Autodesk Inventor part; units mm, degrees
ref_plane "YZ Plane" through (0, 0, 0) normal (1, 0, 0) x (0, 1, 0)
ref_plane "XZ Plane" through (0, 0, 0) normal (0, 1, 0) x (-1, 0, 0)
ref_plane "XY Plane" through (0, 0, 0) normal (0, 0, 1) x (1, 0, 0)
sketch "Sketch1" plane through (0, 0, 0) normal (1, 0, 0) x (0, 1, 0)
  line L0 (0, 0) -> (50.8, 0)
  line L1 (50.8, 0) -> (50.8, -25.4)
  line L2 (50.8, -25.4) -> (0, -25.4)
  line L3 (0, -25.4) -> (0, 0)
  line L4 (2.54, -2.54) -> (48.26, -2.54)
  line L5 (48.26, -2.54) -> (48.26, -22.86)
  line L6 (48.26, -22.86) -> (2.54, -22.86)
  line L7 (2.54, -22.86) -> (2.54, -2.54)
  dimension "d0" = 50.8
  dimension "d1" = 25.4
  dimension "d2" = 45.72
  dimension "d3" = 20.32
  dimension "d4" = 2.54
  dimension "d5" = 2.54
extrude "Extrusion1" add sketch "Sketch1" along normal blind 76.2
sketch "Sketch2" plane through (0, 50.8, 0) normal (0, 1, 0) x (1, 0, 0)
  line L0 (0, 0) -> (0, 25.4)
  line L1 (0, 0) -> (76.2, 0)
  line L2 (76.2, 25.4) -> (76.2, 0)
  line L3 (0, 25.4) -> (76.2, 25.4)
  point P0 (12.7, 12.7)
  point P1 (38.1, 12.7)
  point P2 (63.5, 12.7)
  dimension "d8" = 12.7
  dimension "d9" = 12.7
  dimension "d10" = 12.7
  dimension "d11" = 12.7
  dimension "d12" = 38.1
  dimension "d13" = 63.5
hole "Hole1" at (12.7, 50.8, -12.7) at (38.1, 50.8, -12.7) at (63.5, 50.8, -12.7) direction (0, -1, 0) diameter 3.9688 end through all
sketch "Sketch4" plane through (0, 50.8, 0) normal (0, 1, 0) x (1, 0, 0)
  circle A0 centre (38.1, 12.7) radius 1.9844
  circle A1 centre (12.7, 12.7) radius 1.9844
  circle A2 centre (63.5, 12.7) radius 1.9844
  line L0 (0, 0) -> (0, 25.4)
  line L1 (0, 0) -> (76.2, 0)
  line L2 (76.2, 25.4) -> (76.2, 0)
  line L3 (0, 25.4) -> (76.2, 25.4)
  circle A3 centre (25.4, 12.7) radius 3.175
  circle A4 centre (12.7, 12.7) radius 3.175
  dimension "d25" = 12.7
  dimension "d26" = 25.4
  dimension "d27" = 6.35
  dimension "d28" = 6.35
extrude "Extrusion3" cut sketch "Sketch4" against normal blind 50.8 contours A3 | A4
properties part number "frame_side"
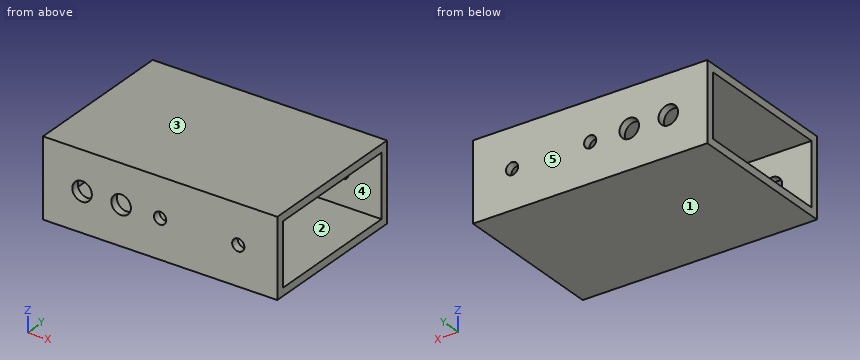
The model under review builds one solid part; all positions refer to its coordinate system, in mm. Face numbers are marked on the shaded views. A direction names the side the tool comes from. Give positions to 0.01 mm unless a question says otherwise; leave off trailing zeros. Write each loop counter-clockwise with the first axis right and the second up, starting at its lowest first coordinate (ties: lowest second). Pieces come first, ordered by that corner, then holes. Notation, with made-up numbers: M 71,-22 L 105,-22 A11 cw 105,-6 Z; hole C -21.5,84.5 d2. An arc over 180 degrees is marked long. Write item = value, one per line. Start each with the question number.
Q1. We need section D-D (x = 63.5). State the section outline as (y, z) points, plus the area to 3 significant figures.
Q2. We need section A-A (y = 12). State the section outline as (x, z) points.
Q3. Mouldability with a two-part tool opening along Y and no side actions: class the marked faces 3, 4 and 5 as released by +Y, released by -Y, zero draft, split by the parting line, or undercut.
Q4. For line 1 (X direction, y = 49.6, z = -12.7) (3 decimals); line 2 (Y direction, x = 34, z = -11.25); line 3 (Z direction, x = 53.5, y = 31), list the stretches that pass through material, from the lowest coordinate up.
Q5. We need section C-C (z = -4.75). State the section outline as (x, y) points.
Q6. We need section B-B (x = 25.4). State the section outline as (y, z) points (3 decimals).
Q7. Machinability: for the marked faces 1 and 2, which of the approach directions +Z, -Z, +X, -X, +Y, -Y give a long, thin tool a straight path to every point of the face, cutting with its end or side? Answer none if there is none.
Q8. Clearance check with a flat-ended pin moving along its axis: pin 1 (12 mm diameter, centred on y = 10, z = -14.5, fed in from +X). State where the tip first meets the part, or that it passes through.
Result set:
q1.outline = M 0,-25.4 L 50.8,-25.4 L 50.8,-14.68 L 48.26,-14.68 L 48.26,-22.86 L 2.54,-22.86 L 2.54,-14.68 L 0,-14.68 Z; M 0,-10.72 L 2.54,-10.72 L 2.54,-2.54 L 48.26,-2.54 L 48.26,-10.72 L 50.8,-10.72 L 50.8,0 L 0,0 Z
q1.area = 341 mm2
q2.outline = M 0,-25.4 L 76.2,-25.4 L 76.2,-22.86 L 0,-22.86 Z; M 0,-2.54 L 76.2,-2.54 L 76.2,0 L 0,0 Z
q3.face_3 = zero draft
q3.face_4 = undercut
q3.face_5 = released by +Y
q4.line_1 = 0 to 9.525, 15.875 to 22.225, 28.575 to 36.116, 40.084 to 61.516, 65.484 to 76.2
q4.line_2 = 0 to 2.54, 48.26 to 50.8
q4.line_3 = -25.4 to -22.86, -2.54 to 0
q5.outline = M 0,0 L 76.2,0 L 76.2,2.54 L 0,2.54 Z; M 0,48.26 L 76.2,48.26 L 76.2,50.8 L 0,50.8 Z
q6.outline = M 0,-25.4 L 50.8,-25.4 L 50.8,-15.875 L 48.26,-15.875 L 48.26,-22.86 L 2.54,-22.86 L 2.54,-15.875 L 0,-15.875 Z; M 0,-9.525 L 2.54,-9.525 L 2.54,-2.54 L 48.26,-2.54 L 48.26,-9.525 L 50.8,-9.525 L 50.8,0 L 0,0 Z
q7.face_1 = -Z, +X, -X, +Y, -Y
q7.face_2 = +X, -X
q8.pin_1 = through
